For this review, use the dimensioned drawing (mm, ordinates from the lowest corner) and the shaded views. Coordinates: 2 decimals unless noted, no trailing zeros. Loops run counter-clockwise (first coordinate to the right, second up) from the corner with the lowest first, then second, coordinate; pieces in that order, holes last. Notation, with made-up numbers: (-17, 60) - (28, 60) arc R27 cw to (28, 79) - close; hole circle Ø8 at (-5, 70). An arc over 180 degrees is marked (long way). Use a Markdown table: item, result. Add a question column.
1) Clearance check with a flat-ended pin moving along its axis: pin 1 (6 mm diameter, centred on x = 53, y = 38.5, fed in from +Z). State where the tip first meets the part, or that it passes through.
2) Add section D-D, the plane y = 19. Give the boundary of the cut face in (x, z), and give its area (3 significant figures).
3) Add section B-B, the plane y = 5. Give the boundary of the cut face in (x, z).
4) Add section A-A, the plane x = 77.5. Give the boundary of the cut face in (y, z).
5) To check wall thickness, follow L1, parallel to Y at x = 77.5, z = 1.95; L2, parallel to Z at x = 18.5, y = 34; L3, parallel to X at y = 21, z = 0.5. State the ranges of each line that lie inside material, in increasing order. Write a range as [from, to].
6) Add section C-C, the plane x = 129. Give the boundary of the cut face in (y, z), and give its area (3 significant figures).
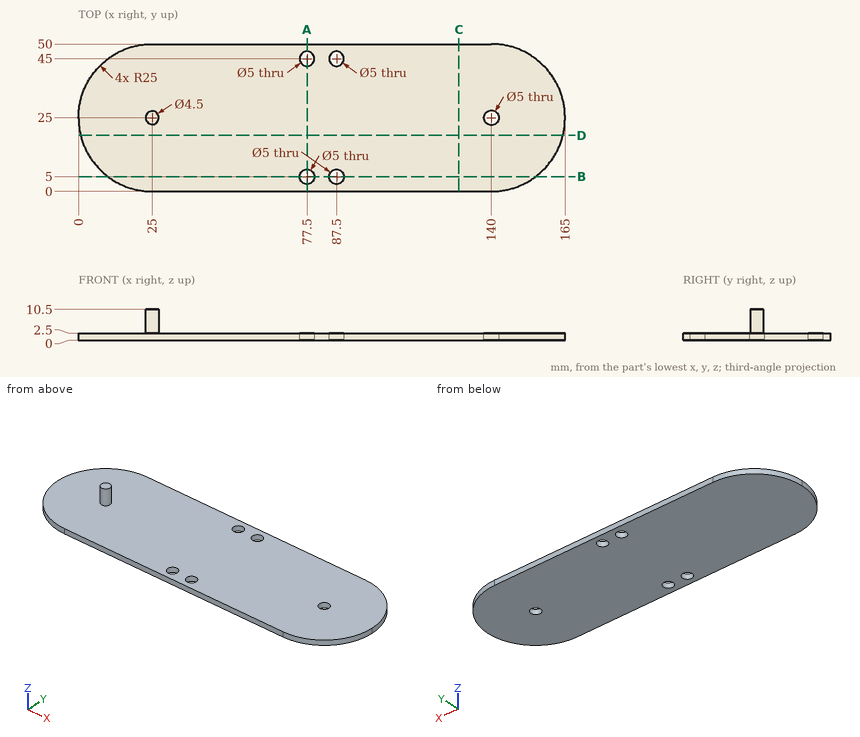
From the geometry:
| question | item | result |
|---|---|---|
| 1 | pin 1 | stops at z = 2.5 |
| 2 | outline | (0.73, 0) - (164.27, 0) - (164.27, 2.5) - (0.73, 2.5) - close |
| 2 | area | 409 mm^2 |
| 3 | outline | (10, 0) - (75, 0) - (75, 2.5) - (10, 2.5) - close; (80, 0) - (85, 0) - (85, 2.5) - (80, 2.5) - close; (90, 0) - (155, 0) - (155, 2.5) - (90, 2.5) - close |
| 4 | outline | (0, 0) - (2.5, 0) - (2.5, 2.5) - (0, 2.5) - close; (7.5, 0) - (42.5, 0) - (42.5, 2.5) - (7.5, 2.5) - close; (47.5, 0) - (50, 0) - (50, 2.5) - (47.5, 2.5) - close |
| 5 | L1 | y = [0, 2.5], [7.5, 42.5], [47.5, 50] |
| 5 | L2 | z = [0, 2.5] |
| 5 | L3 | x = [0.32, 164.68] |
| 6 | outline | (0, 0) - (50, 0) - (50, 2.5) - (0, 2.5) - close |
| 6 | area | 125 mm^2 |
